Verification items for the finished model (mm, model axes). Give positions to 0.01 mm unless a question says otherwise; leave off trailing zeros. Write each loop counter-clockwise with the first axis right and the second up, starting at its lowest first coordinate (ties: lowest second). Pieces come first, ordered by that corner, then holes. Notation, with made-up numbers: (-21, -7) -> (6, -7) arc R7 cw to (6, -1) -> close; hole circle Ø10 at (16, 42.5). An arc over 180 degrees is marked (long way). Answer as CSV lines item,"result". Start each with the question number.
1) Material ranges on L1, parallel to Z at x = 33.55, y = -1.5; L2, parallel to X at y = 1.25, z = 1, recorded low to high.
2) Sectioned sample at C-C on z = 0.75. Record the cut outline in (x, y).
3) Sectioned sample at B-B on x = 4.55. Record the cut outline in (y, z), and give its area (3 significant figures).
4) Sectioned sample at A-A on y = 0. Record the cut outline in (x, z).
5) Mould release check, pull along Z, two halves, no side actions. Record for faces 1 (the flat face through (19, -4.762, 3)), 2 (the flat face through (19, 0, 4.762)), 3 (the cylindrical face through (16.748, -0.067, -0.725)): released by +Z, released by -Z, zero draft, split by the parting line, or undercut.
6) Sectioned sample at D-D on y = 4.25. Record the cut outline in (x, z).
```python
from build123d import *

# Parameters (mm, degrees)
SKETCH1_W              = 9.525
SKETCH1_H              = 9.525
BOSS_EXTRUDE1_DEPTH    = 38.1
F_10_24_TAPPED_HOLE1_D = 4.826
F_10_24_TAPPED_HOLE2_D = 4.826


with BuildPart() as part:
    # Sketch1 → Boss-Extrude1 (new body)
    with BuildSketch(Plane(origin=(0, 0, 0), x_dir=(0, 0, -1), z_dir=(1, 0, 0))):
        Rectangle(SKETCH1_W, SKETCH1_H)
    extrude(amount=BOSS_EXTRUDE1_DEPTH)

    # #10-24 Tapped Hole1 (through all)
    with Locations(Plane(origin=(0, 4.7625, 0), x_dir=(1, 0, 0), z_dir=(0, 1, 0))):
        with Locations((4.55, 0), (19.05, 0), (33.55, 0)):
            Hole(F_10_24_TAPPED_HOLE1_D / 2)

    # #10-24 Tapped Hole2 (through all)
    with Locations(Plane.XY.offset(4.7625)):
        with Locations((11.8, 0), (26.3, 0)):
            Hole(F_10_24_TAPPED_HOLE2_D / 2)


solid = part.part
```
Ans:
1,L1,"z = -4.76 to -2.41, 2.41 to 4.76"
1,L2,"x = 0 to 2.35, 6.75 to 9.74, 13.86 to 16.85, 21.25 to 24.24, 28.36 to 31.35, 35.75 to 38.1"
2,outline,"(0, -4.76) -> (2.26, -4.76) -> (2.26, 4.76) -> (0, 4.76) -> close; (6.84, -4.76) -> (16.76, -4.76) -> (16.76, 4.76) -> (6.84, 4.76) -> close; (21.34, -4.76) -> (31.26, -4.76) -> (31.26, 4.76) -> (21.34, 4.76) -> close; (35.84, -4.76) -> (38.1, -4.76) -> (38.1, 4.76) -> (35.84, 4.76) -> close; hole circle Ø4.83 at (11.8, 0); hole circle Ø4.83 at (26.3, 0)"
3,outline,"(-4.76, -4.76) -> (4.76, -4.76) -> (4.76, -2.41) -> (-4.76, -2.41) -> close; (-4.76, 2.41) -> (4.76, 2.41) -> (4.76, 4.76) -> (-4.76, 4.76) -> close"
3,area,"44.8 mm²"
4,outline,"(0, -4.76) -> (9.39, -4.76) -> (9.39, 4.76) -> (0, 4.76) -> close; (14.21, -4.76) -> (23.89, -4.76) -> (23.89, 4.76) -> (14.21, 4.76) -> close; (28.71, -4.76) -> (38.1, -4.76) -> (38.1, 4.76) -> (28.71, 4.76) -> close; hole circle Ø4.83 at (4.55, 0); hole circle Ø4.83 at (19.05, 0); hole circle Ø4.83 at (33.55, 0)"
5,face 1,"zero draft"
5,face 2,"released by +Z"
5,face 3,"undercut"
6,outline,"(0, -4.76) -> (38.1, -4.76) -> (38.1, 4.76) -> (0, 4.76) -> close; hole circle Ø4.83 at (4.55, 0); hole circle Ø4.83 at (19.05, 0); hole circle Ø4.83 at (33.55, 0)"
